```python
from build123d import *

# Parameters (mm, degrees)
SKETCH1_R           = 4.1
SKETCH1_R_2         = 4
SKETCH1_R_3         = 2.6
BOSS_EXTRUDE1_DEPTH = 10
CUT_EXTRUDE1_START  = -4
CUT_EXTRUDE1_DEPTH  = 4
FILLET1_R           = 2
BOSS_EXTRUDE2_START = -20
SKETCH3_R           = 4
BOSS_EXTRUDE2_DEPTH = 20
FILLET2_R           = 1
SKETCH4_R           = 2.6
BOSS_EXTRUDE3_DEPTH = 15
CUT_EXTRUDE2_REACH  = 78.959
FILLET3_R           = 3
CUT_EXTRUDE3_DEPTH  = 6


with BuildPart() as part:
    # Sketch1 → Boss-Extrude1 (new body)
    with BuildSketch(Plane(origin=(0, 0, 0), x_dir=(1, 0, 0), z_dir=(0, 1, 0))):
        with BuildLine():
            Line((11.273947383, 72.313413723), (4.792068361, 72.313413723))
            Line((4.792068361, 72.313413723), (-53.726052617, 72.313413723))
            ThreePointArc((-53.726052617, 72.313413723), (-57.261586523, 70.848947629), (-58.726052617, 67.313413723))
            Line((-58.726052617, 67.313413723), (-58.726052617, 34.313413723))
            ThreePointArc((-58.726052617, 34.313413723), (-57.261586523, 30.777879817), (-53.726052617, 29.313413723))
            Line((-53.726052617, 29.313413723), (-5.726052617, 29.313413723))
            ThreePointArc((-5.726052617, 29.313413723), (1.345015195, 26.384481534), (4.273947383, 19.313413723))
            Line((4.273947383, 19.313413723), (4.273947383, 17.313413723))
            ThreePointArc((4.273947383, 17.313413723), (5.738413477, 13.777879817), (9.273947383, 12.313413723))
            Line((9.273947383, 12.313413723), (36.273947383, 12.313413723))
            ThreePointArc((36.273947383, 12.313413723), (39.809481289, 13.777879817), (41.273947383, 17.313413723))
            Line((41.273947383, 17.313413723), (41.273947383, 42.313413723))
            ThreePointArc((41.273947383, 42.313413723), (32.487150819, 63.526617158), (11.273947383, 72.313413723))
        make_face()
        with Locations(Location((33.273947383, 20.313413723, 0), (0, 0, 270))):
            Circle(SKETCH1_R, mode=Mode.SUBTRACT)
        with Locations(Location((12.273947383, 20.313413723, 0), (0, 0, 270))):
            Circle(SKETCH1_R_2, mode=Mode.SUBTRACT)
        with Locations(Location((-50.726052617, 64.313413723, 0), (0, 0, 270))):
            Circle(SKETCH1_R_3, mode=Mode.SUBTRACT)
        with Locations(Location((-50.726052617, 37.313413723, 0), (0, 0, 270))):
            Circle(SKETCH1_R_3, mode=Mode.SUBTRACT)
        with BuildLine():
            Line((34.171420048, 34.313413723), (26.134777641, 34.313413723))
            ThreePointArc((26.134777641, 34.313413723), (25.561526201, 34.49403421), (25.19535667, 34.97064815))
            Line((25.19535667, 34.97064815), (14.615821544, 63.966084002))
            ThreePointArc((14.615821544, 63.966084002), (14.998488248, 65.980552022), (16.952543045, 66.601989919))
            ThreePointArc((16.952543045, 66.601989919), (32.892900514, 54.755368869), (35.127730175, 35.021059585))
            ThreePointArc((35.127730175, 35.021059585), (34.766250218, 34.509562325), (34.171420048, 34.313413723))
        make_face(mode=Mode.SUBTRACT)
        with BuildLine():
            Line((-42.557674575, 35.313413723), (-42.557674575, 60.452375226))
            ThreePointArc((-42.557674575, 60.452375226), (-41.891342574, 61.395065879), (-40.780343242, 61.081466633))
            Line((-40.780343242, 61.081466633), (-20.435473581, 35.94250513))
            ThreePointArc((-20.435473581, 35.94250513), (-20.310283056, 34.882769674), (-21.212804914, 34.313413723))
            Line((-21.212804914, 34.313413723), (-41.557674575, 34.313413723))
            ThreePointArc((-41.557674575, 34.313413723), (-42.264781356, 34.606306941), (-42.557674575, 35.313413723))
        make_face(mode=Mode.SUBTRACT)
        with BuildLine():
            Line((-37.245793747, 67.251595954), (5.443945576, 67.251595954))
            ThreePointArc((5.443945576, 67.251595954), (6.346467434, 66.682240002), (6.221276909, 65.622504547))
            Line((6.221276909, 65.622504547), (-15.123592752, 39.247901728))
            ThreePointArc((-15.123592752, 39.247901728), (-15.900924085, 38.876993135), (-16.678255419, 39.247901728))
            Line((-16.678255419, 39.247901728), (-38.02312508, 65.622504547))
            ThreePointArc((-38.02312508, 65.622504547), (-38.148315604, 66.682240002), (-37.245793747, 67.251595954))
        make_face(mode=Mode.SUBTRACT)
        with BuildLine():
            Line((19.622800135, 35.656179295), (10.526467022, 60.58658882))
            ThreePointArc((10.526467022, 60.58658882), (9.751557094, 61.230198488), (8.809714717, 60.872914654))
            Line((8.809714717, 60.872914654), (-11.36637459, 35.94250513))
            ThreePointArc((-11.36637459, 35.94250513), (-11.491565114, 34.882769674), (-10.589043257, 34.313413723))
            Line((-10.589043257, 34.313413723), (18.683379163, 34.313413723))
            ThreePointArc((18.683379163, 34.313413723), (19.502758676, 34.740162282), (19.622800135, 35.656179295))
        make_face(mode=Mode.SUBTRACT)
    extrude(amount=BOSS_EXTRUDE1_DEPTH)

    # Sketch2 → Cut-Extrude1 (cut)
    with BuildSketch(Plane(origin=(0, 10, 0), x_dir=(1, 0, 0), z_dir=(0, 1, 0)).offset(CUT_EXTRUDE1_START)):
        with BuildLine():
            Line((33.273947383, 27.813413723), (41.273947383, 27.813413723))
            Line((41.273947383, 27.813413723), (41.273947383, 17.313413723))
            ThreePointArc((41.273947383, 17.313413723), (39.809481289, 13.777879817), (36.273947383, 12.313413723))
            Line((36.273947383, 12.313413723), (25.773947383, 12.313413723))
            Line((25.773947383, 12.313413723), (25.773947383, 20.313413723))
            ThreePointArc((25.773947383, 20.313413723), (27.970646524, 25.616714582), (33.273947383, 27.813413723))
        make_face()
    extrude(amount=CUT_EXTRUDE1_DEPTH, mode=Mode.SUBTRACT)

    # Fillet1
    fillet1_edges = [part.edges().sort_by_distance(p)[0] for p in [
        (41.273947383, 8, -27.813413723),
        (25.773947383, 8, -12.313413723),
    ]]
    fillet(fillet1_edges, radius=FILLET1_R)

    # Sketch3 → Boss-Extrude2 (add)
    with BuildSketch(Plane(origin=(0, 10, 0), x_dir=(1, 0, 0), z_dir=(0, 1, 0)).offset(BOSS_EXTRUDE2_START)):
        with Locations(Location((12.273947383, 20.313413723, 0), (0, 0, 270))):
            Circle(SKETCH3_R)
    extrude(amount=BOSS_EXTRUDE2_DEPTH)

    # Fillet2
    fillet2_edges = [part.edges().sort_by_distance(p)[0] for p in [
        (12.273947383, -10, -24.313413723),
        (12.273947383, 0, -24.313413723),
    ]]
    fillet(fillet2_edges, radius=FILLET2_R)

    # Sketch4 → Boss-Extrude3 (add)
    with BuildSketch(Plane(origin=(0, 10, 0), x_dir=(1, 0, 0), z_dir=(0, 1, 0))):
        with BuildLine():
            Line((-58.726052617, 67.313413723), (-58.726052617, 34.313413723))
            ThreePointArc((-58.726052617, 34.313413723), (-57.261586523, 30.777879817), (-53.726052617, 29.313413723))
            Line((-53.726052617, 29.313413723), (-5.726052617, 29.313413723))
            Line((-5.726052617, 29.313413723), (-5.726052617, 34.313413723))
            Line((-5.726052617, 34.313413723), (-10.589043257, 34.313413723))
            ThreePointArc((-10.589043257, 34.313413723), (-11.491565114, 34.882769674), (-11.36637459, 35.94250513))
            Line((-11.36637459, 35.94250513), (-5.726052617, 42.91191999))
            Line((-5.726052617, 42.91191999), (-5.726052617, 50.813413723))
            Line((-5.726052617, 50.813413723), (-15.123592752, 39.247901728))
            ThreePointArc((-15.123592752, 39.247901728), (-15.900924085, 38.876993135), (-16.678255419, 39.247901728))
            Line((-16.678255419, 39.247901728), (-38.02312508, 65.622504547))
            ThreePointArc((-38.02312508, 65.622504547), (-38.148315604, 66.682240002), (-37.245793747, 67.251595954))
            Line((-37.245793747, 67.251595954), (-5.726052617, 67.251595954))
            Line((-5.726052617, 67.251595954), (-5.726052617, 72.313413723))
            Line((-5.726052617, 72.313413723), (-53.726052617, 72.313413723))
            ThreePointArc((-53.726052617, 72.313413723), (-57.261586523, 70.848947629), (-58.726052617, 67.313413723))
        make_face()
        with Locations(Location((-50.726052617, 64.313413723, 0), (0, 0, 270))):
            Circle(SKETCH4_R, mode=Mode.SUBTRACT)
        with Locations(Location((-50.726052617, 37.313413723, 0), (0, 0, 270))):
            Circle(SKETCH4_R, mode=Mode.SUBTRACT)
        with BuildLine():
            Line((-40.780343242, 61.081466633), (-20.435473581, 35.94250513))
            ThreePointArc((-20.435473581, 35.94250513), (-20.310283056, 34.882769674), (-21.212804914, 34.313413723))
            Line((-21.212804914, 34.313413723), (-41.557674575, 34.313413723))
            ThreePointArc((-41.557674575, 34.313413723), (-42.264781356, 34.606306941), (-42.557674575, 35.313413723))
            Line((-42.557674575, 35.313413723), (-42.557674575, 60.452375226))
            ThreePointArc((-42.557674575, 60.452375226), (-41.891342574, 61.395065879), (-40.780343242, 61.081466633))
        make_face(mode=Mode.SUBTRACT)
    extrude(amount=BOSS_EXTRUDE3_DEPTH)

    # Sketch5 → Cut-Extrude2 (cut, up to next)
    with BuildSketch(Plane.XY.offset(-29.313413723), mode=Mode.PRIVATE) as cut_extrude2_sk1:
        Polygon((-5.726052617, 10), (-43.726052617, 25), (-5.726052617, 25), align=None)
    cut_extrude2_tool1 = extrude(cut_extrude2_sk1.sketch, amount=-CUT_EXTRUDE2_REACH, mode=Mode.PRIVATE) & part.part
    # Sketch5 → Cut-Extrude2 (cut, up to next)
    with BuildSketch(Plane.XY.offset(-29.313413723), mode=Mode.PRIVATE) as cut_extrude2_sk2:
        Polygon((-53.726052617, 15), (-43.726052617, 15), (-5.726052617, 0), (-60.945305148, 0), (-60.945305148, 15), align=None)
    cut_extrude2_tool2 = extrude(cut_extrude2_sk2.sketch, amount=-CUT_EXTRUDE2_REACH, mode=Mode.PRIVATE) & part.part
    add(cut_extrude2_tool1.solids().sort_by_distance((-18.392719, 20, -29.313414))[0], mode=Mode.SUBTRACT)
    add(cut_extrude2_tool2.solids().sort_by_distance((-41.1745, 6.188543, -29.313414))[0], mode=Mode.SUBTRACT)

    # Fillet3
    fillet3_edges = [part.edges().sort_by_distance(p)[0] for p in [
        (-5.726052617, 10, -31.813413723),
        (-5.726052617, 10, -46.862666856),
        (-5.726052617, 10, -69.782504838),
        (-43.726052617, 15, -50.813413723),
    ]]
    fillet(fillet3_edges, radius=FILLET3_R)
    fillet3_2_edges = [part.edges().sort_by_distance(p)[0] for p in [
        (-5.726052617, 0, -69.782504838),
        (-5.726052617, 0, -46.885905285),
        (-5.726052617, 0, -31.813413723),
        (-43.726052617, 25, -50.813413723),
    ]]
    fillet(fillet3_2_edges, radius=FILLET3_R)

    # Sketch6 → Cut-Extrude3 (cut)
    with BuildSketch(Plane(origin=(0, 15, 0), x_dir=(-1, 0, 0), z_dir=(0, -1, 0))):
        Polygon((54.800383951, 61.902364674), (54.85124801, 66.636363637), (50.776916675, 69.047412686), (46.651721283, 66.724462771), (46.600857225, 61.990463808), (50.675188559, 59.57941476), align=None)
        Polygon((54.801038143, 39.66614114), (50.726023668, 42.018818416), (46.651038143, 39.666090999), (46.651067091, 34.960686305), (50.726081566, 32.608009029), (54.801067091, 34.960736446), align=None)
    extrude(amount=-CUT_EXTRUDE3_DEPTH, mode=Mode.SUBTRACT)


solid = part.part
```
The model under review builds one solid part; all positions refer to its coordinate system, in mm. A direction names the side the tool comes from. Give positions to 0.01 mm unless a question says otherwise; leave off trailing zeros. Write each loop counter-clockwise with the first axis right and the second up, starting at its lowest first coordinate (ties: lowest second). Pieces come first, ordered by that corner, then holes.
(1) For P1, Ø3, axis at y = 8.5, z = -16.5, coming from the +X side; P2, Ø12, axis at y = -5, z = -49, coming from the +X side; P3, Ø13, axis at x = 33.27, z = -20.31, coming from the +Y side, all flat-tipped, find the tip position at first contact; note any pin that passes through.
(2) The part is to be moulded in two halves that separate along Z. For faces 5 (the cylindrical face through (14.98, -5.06, -23.26)), 6 (the cylindrical face through (5.7, 4.93, -13.817)), 7 (the flat face through (-27, 13, -52)), say which applies: released by +Z, released by -Z, zero draft, split by the parting line, or undercut.
(3) Consider section B-B, the plane z = -58. Give the boundary of the cut face in (x, y).
(4) Consider section C-C, the plane y = -4. Give the boundary of the cut face in (x, z), and give its area (3 significant figures).
(5) Consider section D-D, the plane x = -3.5. Give the boundary of the cut face in (y, z).
(6) Consider section A-A, the plane x = -29. Give the boundary of the cut face in (y, z), and give its area (3 significant figures).
(7) Tool access review of faces 1 (the flat face through (-48.74, 17.96, -67.9)), 2 (the flat face through (-51, 15, -51)), 3 (the cylindrical face through (32.75, 4.93, -55)), 4 (the flat face through (4.274, 5, -18)): name each direction out of +Z, -Z, +X, -X, +Y, -Y from which nothing blocks a thin tool from reaching the whole face with its end or side.
(8) To check wall thickness, follow L1, parallel to X at y = 1, z = -61; L2, parallel to X at y = 3.5, z = -44.5; L3, parallel to Y at x = 13.5, z = -70. State the ranges of each line that lie inside material, in increasing order.
Returned:
1. P1: stops at x = 25.77
1. P2: stops at x = 41.08
1. P3: stops at y = 6
2. face 5: split by the parting line
2. face 6: released by +Z
2. face 7: undercut
3. outline: (-58.73, 15) - (-44.3, 15) arc R3 cw to (-43.2, 14.79) - (-42.56, 14.54) - (-42.56, 24.54) - (-43.2, 24.79) arc R3 ccw to (-44.3, 25) - (-58.73, 25) - close; (-38.29, 12.85) - (-31.85, 10.31) - (-31.85, 20.31) - (-38.29, 22.85) - close; (0.05, 0) - (6.48, 0) - (6.48, 10) - (0.05, 10) - close; (11.47, 0) - (16.79, 0) - (16.79, 10) - (11.47, 10) - close; (30.67, 0) - (36.85, 0) - (36.85, 10) - (30.67, 10) - close
4. outline: circle Ø8 at (12.27, -20.31)
4. area: 50.3 mm2
5. outline: (0, -72.31) - (10, -72.31) - (10, -67.25) - (0, -67.25) - close; (0, -53.61) - (10, -53.61) - (10, -45.66) - (0, -45.66) - close; (0, -34.31) - (10, -34.31) - (10, -29.06) - (0, -29.06) - close
6. outline: (9.19, -72.31) - (19.19, -72.31) - (19.19, -67.25) - (9.19, -67.25) - close; (9.19, -54.47) - (19.19, -54.47) - (19.19, -46.53) - (9.19, -46.53) - close; (9.19, -34.31) - (19.19, -34.31) - (19.19, -29.31) - (9.19, -29.31) - close
6. area: 180 mm2
7. face 1: -Y
7. face 2: +Z, -Z, -X, -Y
7. face 3: +Y, -Y
7. face 4: +Z, -X, +Y, -Y
8. L1: x = 2.48 to 8.93, 10.24 to 15.7, 27.8 to 34.74
8. L2: x = -10.87 to -4.44, 16.4 to 21.72, 36.12 to 41.19
8. L3: y = 0 to 10
